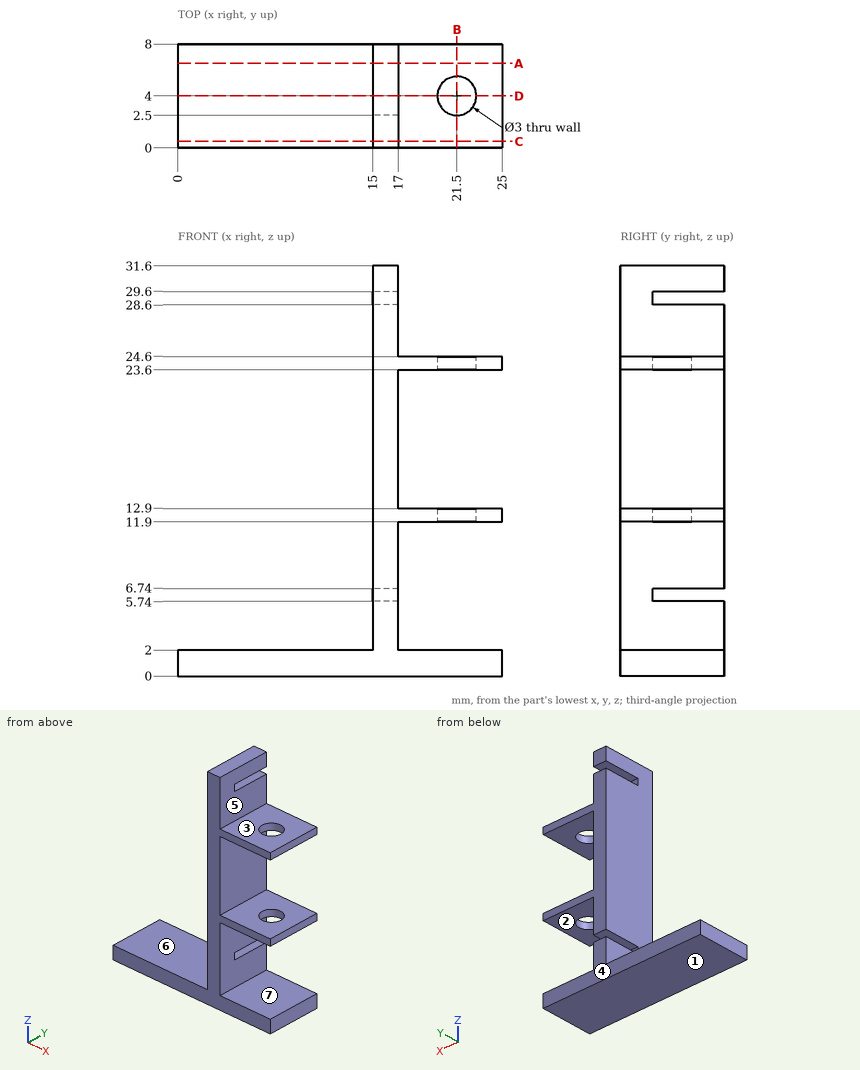
The drawing under review shows one solid part. Ordinate dimensions are in mm from its lowest x, y, z. A direction names the side the tool comes from. Give positions to 0.01 mm unless a question says otherwise; leave off trailing zeros. Loops run counter-clockwise (first coordinate to the right, second up) from the corner with the lowest first, then second, coordinate; pieces in that order, holes last. Notation, with made-up numbers: M 47.5,-18.5 L 80.5,-18.5 A17 ccw 80.5,-6.5 Z; hole C 46.5,-28 d10. An arc over 180 degrees is marked long. Return JSON: item names as keys, results as strings. Group by question number.
Item 1: We need section A-A (y = 6.5). Give the boundary of the cut face in (x, z).
Item 2: Mouldability with a two-part tool opening along Z and no side actions: class the marked faces 1, 2, 3 and 4 as released by +Z, released by -Z, zero draft, split by the parting line, or undercut.
Item 3: Insertion check: pin 1 Ø2.5 at (y, z) = (4, 18) entering from +X; pin 2 Ø2.5 at (x, y) = (20, 3) entering from +Z; pin 3 Ø4 at (x, z) = (21.5, 9) entering from -Y; pin 4 Ø1 at (y, z) = (5.5, 13) entering from -X. Each pin has a flat end and moves straight along its axis. Give the tip position at first contact, or say it passes through.
Item 4: Tool access review of the marked faces 5, 6 and 7: name each direction out of +Z, -Z, +X, -X, +Y, -Y from which nothing blocks a thin tool from reaching the whole face with its end or side.
Item 5: We need section D-D (y = 4). Give the number of separate pieces and of enclosed holes in the cut face, and give its area (3 significant figures).
Item 6: For probe 1 along Y at (x, z) = (21.5, 24.3); probe 2 along X at (y, z) = (4, 12.2); probe 3 along Z at (x, y) = (22, 6), list the stretches that pass through material, from the lowest coordinate up.
Item 7: We need section B-B (x = 21.5). Give the boundary of the cut face in (y, z), and give its area (3 significant figures).
Item 8: We need section C-C (y = 0.5). Give the boundary of the cut face in (x, z).
Output:
{
 "1": {"outline": "M 0,0 L 25,0 L 25,2 L 17,2 L 17,5.74 L 15,5.74 L 15,2 L 0,2 Z; M 15,6.74 L 17,6.74 L 17,11.9 L 25,11.9 L 25,12.9 L 17,12.9 L 17,23.6 L 25,23.6 L 25,24.6 L 17,24.6 L 17,28.6 L 15,28.6 Z; M 15,29.6 L 17,29.6 L 17,31.6 L 15,31.6 Z"},
 "2": {"face 1": "released by -Z", "face 2": "undercut", "face 3": "released by +Z", "face 4": "zero draft"},
 "3": {"pin 1": "stops at x = 17", "pin 2": "stops at z = 24.6", "pin 3": "passes through", "pin 4": "stops at x = 15"},
 "4": {"face 5": "+Z, +X, +Y, -Y", "face 6": "+Z, -X, +Y, -Y", "face 7": "+X, +Y, -Y"},
 "5": {"separate pieces": "5", "enclosed holes": "0", "area": "115 mm^2"},
 "6": {"probe 1": "y = 0 to 2.5, 5.5 to 8", "probe 2": "x = 15 to 20, 23 to 25", "probe 3": "z = 0 to 2, 11.9 to 12.9, 23.6 to 24.6"},
 "7": {"outline": "M 0,0 L 8,0 L 8,2 L 0,2 Z; M 0,11.9 L 2.5,11.9 L 2.5,12.9 L 0,12.9 Z; M 0,23.6 L 2.5,23.6 L 2.5,24.6 L 0,24.6 Z; M 5.5,11.9 L 8,11.9 L 8,12.9 L 5.5,12.9 Z; M 5.5,23.6 L 8,23.6 L 8,24.6 L 5.5,24.6 Z", "area": "26.0 mm^2"},
 "8": {"outline": "M 0,0 L 25,0 L 25,2 L 17,2 L 17,11.9 L 25,11.9 L 25,12.9 L 17,12.9 L 17,23.6 L 25,23.6 L 25,24.6 L 17,24.6 L 17,31.6 L 15,31.6 L 15,2 L 0,2 Z"}
}
